Build history of the part. All positions in model axes, mm. A direction names the side the tool comes from. Round coordinates to 2 decimals unless told otherwise and drop trailing zeros. Write each loop counter-clockwise with the first axis right and the second up, starting at its lowest first coordinate (ties: lowest second). Pieces come first, ordered by that corner, then holes. Notation, with made-up numbers: (4, 14.25) - (10, 14.25) arc R16 ccw to (10, 27.25) - close; hole circle Ø11 at (-23, -18.75). An arc over 180 degrees is marked (long way). Answer as a JSON object with one key per item and string values. Group by question number.
Item 1: Flat gauge pins, fed straight in: pin 1 (6 mm diameter, centred on x = -20, y = 7.5, fed in from +Z); pin 2 (3 mm diameter, centred on y = 16.5, z = 3, fed in from -X); pin 3 (3 mm diameter, centred on y = 14, z = 2, fed in from -X). Where does each tip first touch, or does it go through?
Item 2: Which spindle directions (+Z, -Z, +X, -X, +Y, -Y) get a long thin tool onto all of the face, cutting with end or side? Do faces 4 (the flat face through (6, -21.308, 1)), 5 (the flat face through (-41.849, -8, 1)), 6 (the flat face through (-19, 21.812, 1)), 7 (the flat face through (-1, 1, 2)), 8 (the flat face through (27, 21.812, 1)). Say none if no direction does.
Item 3: Slice it at D-D, the plane y = -14. List the corners of the cut face in (x, z).
Item 4: Slice it at A-A, the plane y = 7.5. List the corners of the cut face in (x, z).
Item 5: Two-plate mould, pull along X, no slides. Class faces 1 (the cylindrical face through (-22, 6, 1)), 2 (the flat face through (-1, 1, 0)), 3 (the cylindrical face through (24.43, -9.12, 3.73)): +X half, -X half, draft (parallel to the pull), parting line (faces both ways), or undercut.
Item 6: Slice it at C-C, the plane x = 10. List the corners of the cut face in (y, z), then the cut area to 3 significant figures.
Item 7: Slice it at B-B, the plane z = 3.2. List the corners of the cut face in (x, y).
Item 8: Probe line 1 (Y direction, x = -20, z = 1.05); line 2 (Y direction, x = 4.5, z = 1.4); line 3 (X direction, y = -14, z = 0.6). List the from-to ranges inside material, lowest first. Write a range as from..to.
from build123d import *

# Parameters (mm, degrees)
SKETCH_1_R          = 2.5
EXTRUDE_1_DEPTH     = 2
SKETCH_2_R          = 5
SKETCH_2_R_2        = 2.5
EXTRUDE_3_DEPTH     = 3.5
CUT_EXTRUDE_1_REACH = 52.835
SKETCH_2_2_R        = 2.5


with BuildPart() as part:
    # Sketch 1 → Extrude 1 (new body)
    with BuildSketch(Plane.XY):
        Polygon((-6.486435689, -27.5), (-0.294279728, -21.307844039), (11.756387017, -21.307844039), (17.948542978, -27.5), (41.84943397, -27.5), (41.84943397, 13.941912539), (33.979452522, 21.811893988), (18.854924629, 21.811893988), (12.020959992, 28.645858624), (-0.811850652, 28.645858624), (-7.645815288, 21.811893988), (-30.698580055, 21.811893988), (-41.84943397, 10.661040072), (-41.84943397, -27.5), align=None)
        with Locations((-20, 7.5)):
            Circle(SKETCH_1_R, mode=Mode.SUBTRACT)
        with Locations((4.5, 23)):
            Circle(SKETCH_1_R, mode=Mode.SUBTRACT)
        with Locations((10, -1.5)):
            Circle(SKETCH_1_R, mode=Mode.SUBTRACT)
    extrude(amount=EXTRUDE_1_DEPTH)

    # Sketch 2 → Extrude 3 (add)
    # profile 1 of 2: a face of its own
    with BuildSketch(Plane.XY.offset(2)):
        with Locations(Location((-32.84943397, -2.5, 0), (0, 0, 180))):
            Circle(SKETCH_2_R)
        with Locations((-32.84943397, -2.5)):
            Circle(SKETCH_2_R_2, mode=Mode.SUBTRACT)
    # profile 2 of 2: a face of its own
    with BuildSketch(Plane.XY.offset(2)):
        with Locations(Location((23.34943397, -14, 0), (0, 0, 180))):
            Circle(SKETCH_2_R)
        with Locations((23.34943397, -14)):
            Circle(SKETCH_2_R_2, mode=Mode.SUBTRACT)
    extrude(amount=EXTRUDE_3_DEPTH)

    # Sketch 2_2 → Cut-Extrude 1 (cut, up to next)
    with BuildSketch(Plane.XY.offset(2), mode=Mode.PRIVATE) as cut_extrude_1_sk1:
        with Locations(Location((-32.84943397, -2.5, 0), (0, 0, 180))):
            Circle(SKETCH_2_2_R)
    cut_extrude_1_tool1 = extrude(cut_extrude_1_sk1.sketch, amount=-CUT_EXTRUDE_1_REACH, mode=Mode.PRIVATE) & part.part
    # Sketch 2_2 → Cut-Extrude 1 (cut, up to next)
    with BuildSketch(Plane.XY.offset(2), mode=Mode.PRIVATE) as cut_extrude_1_sk2:
        with Locations(Location((23.34943397, -14, 0), (0, 0, 180))):
            Circle(SKETCH_2_2_R)
    cut_extrude_1_tool2 = extrude(cut_extrude_1_sk2.sketch, amount=-CUT_EXTRUDE_1_REACH, mode=Mode.PRIVATE) & part.part
    add(cut_extrude_1_tool1.solids().sort_by_distance((-32.849434, -2.5, 2))[0], mode=Mode.SUBTRACT)
    add(cut_extrude_1_tool2.solids().sort_by_distance((23.349434, -14, 2))[0], mode=Mode.SUBTRACT)


solid = part.part
Geometry says:
{
 "1": {"pin 1": "stops at z = 2", "pin 2": "stops at x = -37.13", "pin 3": "stops at x = -40.01"},
 "2": {"face 4": "+Z, -Z, -Y", "face 5": "+Z, -Z, -X, +Y, -Y", "face 6": "+Z, -Z, -X, +Y", "face 7": "+Z", "face 8": "+Z, -Z, +X, +Y"},
 "3": {"outline": "(-41.85, 0) - (20.85, 0) - (20.85, 5.5) - (18.35, 5.5) - (18.35, 2) - (-41.85, 2) - close; (25.85, 0) - (41.85, 0) - (41.85, 2) - (28.35, 2) - (28.35, 5.5) - (25.85, 5.5) - close"},
 "4": {"outline": "(-41.85, 0) - (-22.5, 0) - (-22.5, 2) - (-41.85, 2) - close; (-17.5, 0) - (41.85, 0) - (41.85, 2) - (-17.5, 2) - close"},
 "5": {"face 1": "undercut", "face 2": "draft", "face 3": "parting line"},
 "6": {"outline": "(-21.31, 0) - (-4, 0) - (-4, 2) - (-21.31, 2) - close; (1, 0) - (28.65, 0) - (28.65, 2) - (1, 2) - close", "area": "89.9 mm^2"},
 "7": {"outline": "circle Ø10 at (-32.85, -2.5); circle Ø10 at (23.35, -14); hole circle Ø5 at (-32.85, -2.5); hole circle Ø5 at (23.35, -14)"},
 "8": {"line 1": "y = -27.5..5, 10..21.81", "line 2": "y = -21.31..20.5, 25.5..28.65", "line 3": "x = -41.85..20.85, 25.85..41.85"}
}
